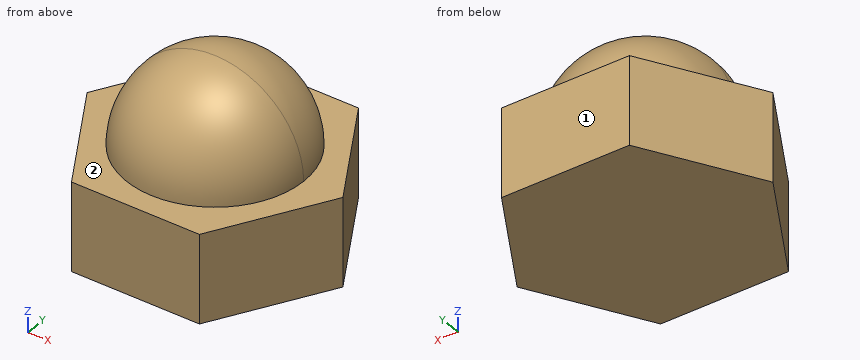
```python
from build123d import *
from build123d import SkipClean  # not in build123d's __all__

# Parameters (mm, degrees)
F1_DEPTH = 4


with BuildPart() as f1:
    # F0 (on Top) → F1 (new body)
    with BuildSketch(Plane.XY):
        Polygon((2.8867513459, 5), (-2.8867513459, 5), (-5.7735026919, 0), (-2.8867513459, -5), (2.8867513459, -5), (5.7735026919, 0), align=None)
    extrude(amount=F1_DEPTH)

    # F2 (on Front) → F3 (revolve)
    with BuildSketch(Plane.XZ):
        with BuildLine():
            Line((-3.9975453725, 4), (4.0024546275, 4))
            ThreePointArc((4.0024546275, 4), (0.0024546275, 8), (-3.9975453725, 4))
        make_face()
    with SkipClean():  # cleaning this boolean's faces spoils the solid; the shape is the same uncleaned
        revolve(axis=Axis((0.0024546275, 0, 4), (1, 0, 0)))


solid = f1.part
```
Input: part model. Units: mm. Frame: model coordinates. Face numbers are marked on the shaded views. A direction names the side the tool comes from. Coordinates: 2 decimals unless noted, no trailing zeros. Loops run counter-clockwise (first coordinate to the right, second up) from the corner with the lowest first, then second, coordinate; pieces in that order, holes last. Notation, with made-up numbers: M 66.5,-10.5 L 98.5,-10.5 A21 cw 98.5,28.5 Z; hole C 53.25,67 d10. An arc over 180 degrees is marked long. Use a Markdown table: item, result. Add a question column.
1) Section D-D, the plane z = 5.75. Return the cut outline in (x, y).
2) Section C-C, the plane x = 4.25. Return the cut outline in (y, z).
3) Line query: L1, parallel to Z at x = 4, y = 1; L2, parallel to X at y = 4, z = 2; L3, parallel to Y at x = -1.5, z = 4.25. Output: solid intervals per line, ascending. Write a range as from..to.
4) Section A-A, the plane x = 0. Return the cut outline in (y, z).
5) Set-up query: the marked faces 1 and 2. Return all of +Z, -Z, +X, -X, +Y, -Y with unobstructed straight access to the full face (end or side cutting, diameter ignored); none if empty.
6) Pin query (flat end, axial travel): P1, Ø5, axis at x = 2.5, y = -2, coming from the +Z side; P2, Ø1.5, axis at x = -4, z = 5, coming from the -Y side. Return the tip coordinate at first contact, or that it passes through.
7) Section B-B, the plane z = 1.75. Return the cut outline in (x, y), plus the area to 3 significant figures.
Answer below:
| question | item | result |
|---|---|---|
| 1 | outline | C 0,0 d7.19 |
| 2 | outline | M -2.64,0 L 2.64,0 L 2.64,4 L -2.64,4 Z |
| 3 | L1 | 0..4 |
| 3 | L2 | -3.46..3.46 |
| 3 | L3 | -3.7..3.7 |
| 4 | outline | M -5,0 L 5,0 L 5,4 L 4,4 A4 ccw -4,4 L -5,4 Z |
| 5 | face 1 | +Z, -Z, +X, -X, +Y |
| 5 | face 2 | +Z |
| 6 | P1 | z = 7.94 |
| 6 | P2 | y = -2.15 |
| 7 | outline | M -5.77,0 L -2.89,-5 L 2.89,-5 L 5.77,0 L 2.89,5 L -2.89,5 Z |
| 7 | area | 86.6 mm2 |
